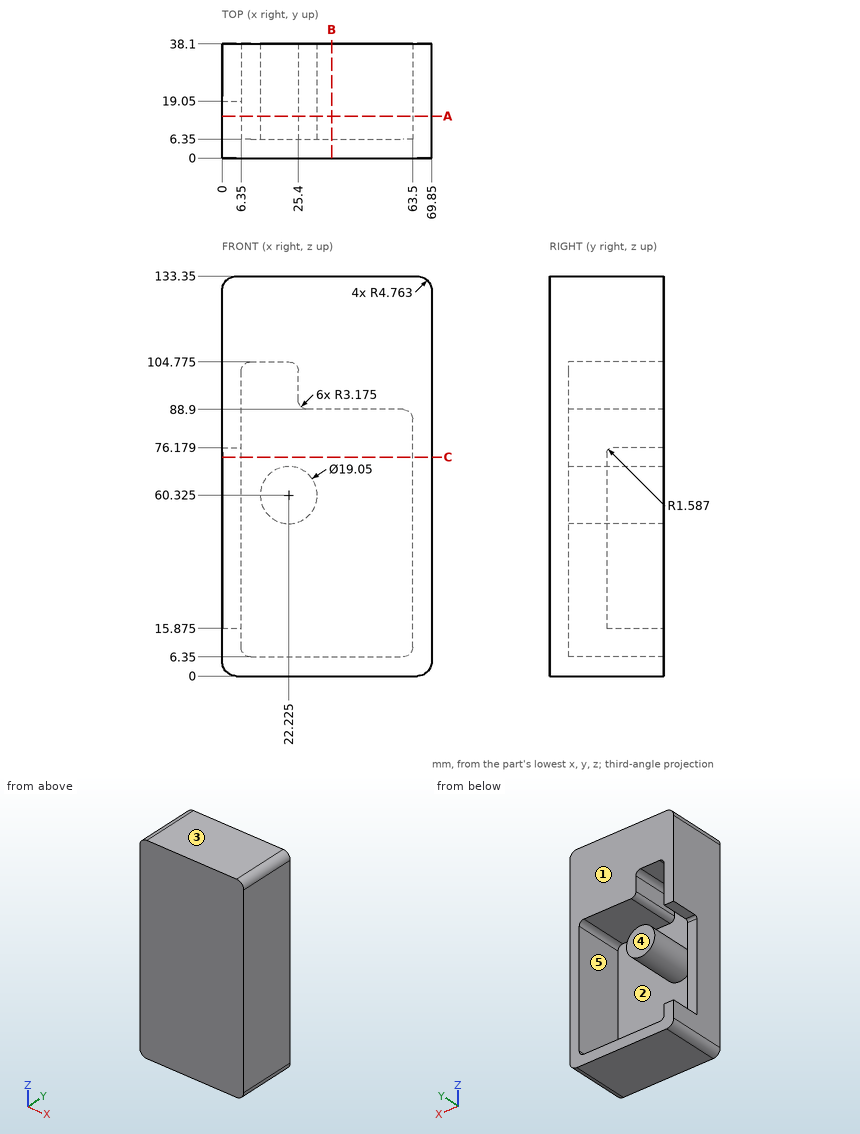
For this review, use the dimensioned drawing (mm, ordinates from the lowest corner) and the shaded views. A direction names the side the tool comes from. Give positions to 0.01 mm unless a question says otherwise; leave off trailing zeros. Loops run counter-clockwise (first coordinate to the right, second up) from the corner with the lowest first, then second, coordinate; pieces in that order, holes last. Notation, with made-up numbers: (-3.75, 39) -> (12.25, 39) arc R17 cw to (12.25, 51) -> close; hole circle Ø8 at (61, 83). An arc over 180 degrees is marked (long way). One line per question, with ' | ' between items. Start each with the question number.
(1) We need section C-C (z = 73). State the section outline as (x, y) points.
(2) For line 1 (Z direction, x = 56, y = 16); line 2 (X direction, y = 13, z = 77); line 3 (X direction, y = 34, z = 101), list the stretches that pass through material, from the lowest coordinate up.
(3) We need section B-B (x = 36.5). State the section outline as (y, z) points.
(4) Insertion check: P1, Ø2, axis at x = 8.5, z = 77, coming from the +Y side; P2, Ø10, axis at x = 61.5, z = 39.5, coming from the +Y side; P3, Ø1.9, axis at x = 1.5, y = 32.5, coming from the -Z side; P4, Ø1.9, axis at x = 3.5, z = 57, coming from the +Y side. Each pin has a flat end and moves straight along its axis. Give the tip position at first contact, or say it passes through.
(5) For the marked faces 4 and 5, list the 3-axis set-ups (+Z, -Z, +X, -X, +Y, -Y) from which the entire face can be reached by the end or side of a thin tool; tool diameter is ignored.
(6) Draft analysis for pull direction Z (two halves, no side actions). For the marked faces 1, 2 and 3, state which applies: +Z half, -Z half, draft (parallel to the pull), parting line (faces both ways), or undercut.
(7) We need section A-A (y = 14). State how many separate pieces and enclosed holes the cut face has, and give its area (3 significant figures).
The answers:
1) outline: (0, 0) -> (69.85, 0) -> (69.85, 38.1) -> (63.5, 38.1) -> (63.5, 6.35) -> (6.35, 6.35) -> (6.35, 19.05) -> (0, 19.05) -> close
2) line 1: z = 0 to 6.35, 88.9 to 133.35 | line 2: x = 0 to 6.35, 63.5 to 69.85 | line 3: x = 0 to 6.35, 25.4 to 69.85
3) outline: (0, 0) -> (38.1, 0) -> (38.1, 6.35) -> (6.35, 6.35) -> (6.35, 88.9) -> (38.1, 88.9) -> (38.1, 133.35) -> (0, 133.35) -> close
4) P1: stops at y = 6.35 | P2: stops at y = 38.1 | P3: stops at z = 0.6 | P4: stops at y = 19.05
5) face 4: +Z, -Z, +X, -X, +Y | face 5: +Y
6) face 1: draft | face 2: undercut | face 3: +Z half
7) separate pieces: 2 | enclosed holes: 1 | area: 4,570 mm^2
